from build123d import *

# Parameters (mm, degrees)
F0_R     = 1.6
F1_DEPTH = 20.7


with BuildPart() as f1:
    # F0 (on Front) → F1 (new body)
    with BuildSketch(Plane.XZ):
        Polygon((163, 0), (158, 5), (158, -18), (163, -13), align=None)
        Polygon((158, -18), (158, 5), (-56, 5), (-72.5, 21.5), (-72.5, 91.5), (-92.5, 91.5), (-92.5, 74.5), (-101.464466, 74.5), (-105, 70.964466), (-105, -14.464466), (-101.464466, -18), align=None)
        with Locations((-100, 0)):
            Circle(F0_R, mode=Mode.SUBTRACT)
        Circle(F0_R, mode=Mode.SUBTRACT)
        with Locations((-100, 36.5)):
            Circle(F0_R, mode=Mode.SUBTRACT)
        with Locations((107, 0)):
            Circle(F0_R, mode=Mode.SUBTRACT)
        with Locations((-100, 66.5)):
            Circle(F0_R, mode=Mode.SUBTRACT)
    extrude(amount=F1_DEPTH)


solid = f1.part
For this review, take the finished solid that the model builds, in its own axes (mm). A direction names the side the tool comes from. Coordinates: 2 decimals unless noted, no trailing zeros. Order: outer loops, then holes, each group sorted by start corner. A loop starts at its lowest first (then second) coordinate and runs counter-clockwise, first axis right, second up. Notation, with made-up numbers: (81, 25) -> (139, 25) arc R31 cw to (139, 51) -> close; hole circle Ø11 at (32.25, 75). An arc over 180 degrees is marked (long way). Return JSON: item names as keys, results as strings.
1. For pin 1 Ø10 at (y, z) = (-4, 74.5) entering from +X; pin 2 Ø10.5 at (x, y) = (12.5, -8.5) entering from +Z; pin 3 Ø4.5 at (x, y) = (-97, -14.5) entering from +Z, all flat-tipped, find the tip position at first contact; note any pin that passes through.
Answer block:
{"pin 1": "x = -72.5", "pin 2": "z = 5", "pin 3": "z = 74.5"}
2. For line 1 (Z direction, x = -100, y = -5.5); line 2 (Z direction, x = 107, y = -10.5); line 3 (X direction, y = -7, z = 66.5), list the stretches that pass through material, from the lowest coordinate up. Write a range as from..to.
Answer block:
{"line 1": "-18..-1.6, 1.6..34.9, 38.1..64.9, 68.1..74.5", "line 2": "-18..-1.6, 1.6..5", "line 3": "-105..-101.6, -98.4..-72.5"}
3. We need section B-B on x = -25.5. Write out the cut boundary in (y, z).
Answer block:
{"outline": "(-20.7, -18) -> (0, -18) -> (0, 5) -> (-20.7, 5) -> close"}
4. We need section A-A on y = -13.75. Write out the cut boundary in (x, z), and give its area (3 significant figures).
Answer block:
{"outline": "(-105, -14.46) -> (-101.46, -18) -> (158, -18) -> (163, -13) -> (163, 0) -> (158, 5) -> (-56, 5) -> (-72.5, 21.5) -> (-72.5, 91.5) -> (-92.5, 91.5) -> (-92.5, 74.5) -> (-101.46, 74.5) -> (-105, 70.96) -> close; hole circle Ø3.2 at (-100, 0); hole circle Ø3.2 at (-100, 36.5); hole circle Ø3.2 at (-100, 66.5); hole circle Ø3.2 at (0, 0); hole circle Ø3.2 at (107, 0)", "area": "8,820 mm²"}
5. Machinability: for faces 1 (the flat face through (52, -10, 5)), 2 (the flat face through (160, -10, -16)), 3 (the flat face through (-92.5, -10, 83)), which of the approach directions +Z, -Z, +X, -X, +Y, -Y give a long, thin tool a straight path to every point of the face, cutting with its end or side? Answer none if there is none.
Answer block:
{"face 1": "+Z, +X, +Y, -Y", "face 2": "-Z, +X, +Y, -Y", "face 3": "+Z, -X, +Y, -Y"}
6. We need section C-C on z = 12. Write out the cut boundary in (x, y).
Answer block:
{"outline": "(-105, -20.7) -> (-63, -20.7) -> (-63, 0) -> (-105, 0) -> close"}
